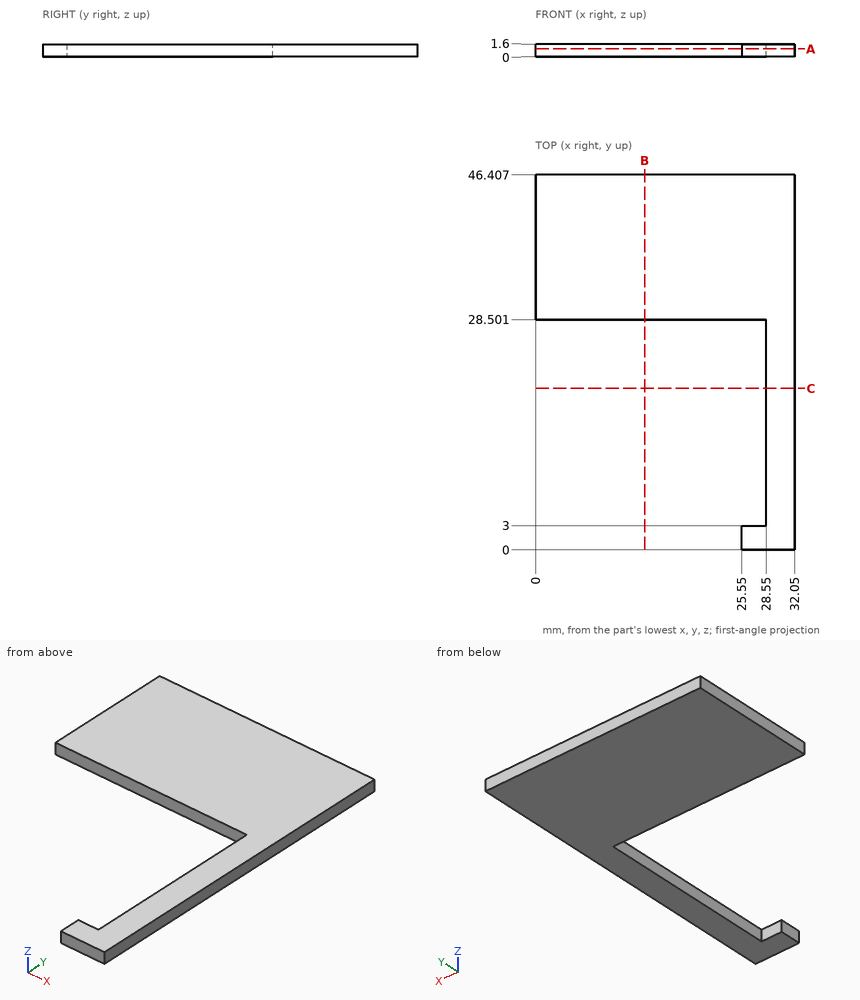
Print and shaded views of the part. All mm, measured from the part's lowest x, y and z. Coordinates: 2 decimals unless noted, no trailing zeros. Loops run counter-clockwise (first coordinate to the right, second up) from the corner with the lowest first, then second, coordinate; pieces in that order, holes last. Notation, with made-up numbers: (54, 78) -> (93, 78) arc R28 cw to (93, 112) -> close; hole circle Ø10 at (82.5, 63.5). An arc over 180 degrees is marked (long way). Use one line per item in the form item = value. Start each with the question number.
(1) Flat gauge pin, fed straight in: pin 1 (10 mm diameter, centred on x = 10, y = 22, fed in from -Z). Where does the tip first touch, or does it go through?
(2) Cut at B-B on x = 13.5. Give the cut face in (y, z).
(3) Probe probe 1 along Y at (x, z) = (6.5, 1.2); probe 2 along Y at (x, z) = (27, 0.65); probe 3 along X at (y, z) = (25.5, 0.7). List the from-to ranges inside material, lowest first. Write a range as from..to.
(4) Cut at A-A on z = 1. Give the cut face in (x, y).
(5) Cut at C-C on y = 20. Give the cut face in (x, z).
Values:
q1.pin_1 = through
q2.outline = (28.5, 0) -> (46.41, 0) -> (46.41, 1.6) -> (28.5, 1.6) -> close
q3.probe_1 = 28.5..46.41
q3.probe_2 = 0..3, 28.5..46.41
q3.probe_3 = 28.55..32.05
q4.outline = (0, 28.5) -> (28.55, 28.5) -> (28.55, 3) -> (25.55, 3) -> (25.55, 0) -> (32.05, 0) -> (32.05, 46.41) -> (0, 46.41) -> close
q5.outline = (28.55, 0) -> (32.05, 0) -> (32.05, 1.6) -> (28.55, 1.6) -> close
